Check sheet for the modelled part. Datum: model origin and axes. Units: mm. A direction names the side the tool comes from. Give positions to 0.01 mm unless a question says otherwise; leave off trailing zeros. Order: outer loops, then holes, each group sorted by start corner. A loop starts at its lowest first (then second) coordinate and runs counter-clockwise, first axis right, second up.
Item 1: Access from +Z, -Z, +X, -X, +Y, -Y to the whole of each face (thin tool, end or side, straight path). Record for faces 4 (the cylindrical face through (889.127, 47.139, -61.478)), 5 (the cylindrical face through (884.46, -24.22, 76.92)).
Item 2: Sectioned sample at A-A on x = 840. Record the boundary of the cut face in (y, z) (3 decimals).
Item 3: Release check for a two-part mould opening along Z. For faces 1 (the conical face through (109.73, 12.52, -2.78)), 2 (the flat face through (95.684, 9, 9)), 3 (the conical face through (1042.485, 75.822, -16.837)) record: released by +Z, released by -Z, zero draft, split by the parting line, or undercut.
Item 4: Gauge pin test, flat ends, axial feed: P1, Ø2, axis at x = 698.5, y = -44.5, coming from the -Z side; P2, Ø1.5, axis at x = 402, z = 34.5, coming from the +Y side; P3, Ø1.5, axis at x = 945.5, y = 62.5, coming from the -Z side. Record the tip position at first contact, or that the pin passes through.
Item 5: Material ranges on line 1 along Y through (x, z) = (861, 0) (3 decimals); line 2 along Z through (x, y) = (686, 61); line 3 along Y through (x, z) = (547.5, -42), recorded low to high.
from build123d import *

# Parameters (mm, degrees)
CHAMFER1_SIZE      = 16.51
SKETCH2_R          = 12.25
CUT_EXTRUDE1_DEPTH = 165


with BuildPart() as part:
    # Sketch1 → Revolve5 (revolve)
    with BuildSketch(Plane(origin=(0, 0, 0), x_dir=(1, 0, 0), z_dir=(0, 1, 0)), mode=Mode.PRIVATE) as revolve5_sk:
        with BuildLine():
            Line((98.225852671, 21.465396338), (95.684220755, 21.057997163))
            Line((95.684220755, 21.057997163), (95.684220755, 0))
            Line((95.684220755, 0), (98.726886962, 0))
            Line((98.726886962, 0), (98.726886962, 18.330178699))
            add(Edge.make_bspline(
                [(98.726886962, 18.330178699), (113.994878644, 20.770132881), (144.577764754, 25.330670583), (205.898051252, 33.589807316), (282.72017046, 42.680521232), (375.073984944, 52.176751592), (467.547747058, 60.469235877), (560.11629344, 67.637393605), (637.322841402, 72.653277734), (694.420933949, 75.753057643), (720.626011218, 76.995143626), (731.378470364, 77.47)],
                knots=[0.119456002, 0.119456002, 0.119456002, 0.119456002, 0.174490002, 0.229524002, 0.339592002, 0.449660001, 0.559728001, 0.669796001, 0.779864001, 0.834898, 0.873185267, 0.873185267, 0.873185267, 0.873185267], degree=3))
            Line((731.378470364, 77.47), (1042.519676327, 77.47))
            Line((1042.519676327, 77.47), (1041.959838164, 80.645))
            Line((1041.959838164, 80.645), (731.308396413, 80.645))
            add(Edge.make_bspline(
                [(98.225852671, 21.465396338), (124.397667511, 25.647873666), (176.884669485, 33.109736653), (282.119502984, 46.013248572), (413.979840243, 59.356838077), (572.506921448, 72.05625987), (678.351858694, 78.306302486), (731.308396413, 80.645)],
                knots=[0.119456002, 0.119456002, 0.119456002, 0.119456002, 0.213682547, 0.307909091, 0.496362181, 0.68481527, 0.873268359, 0.873268359, 0.873268359, 0.873268359], degree=3))
        make_face()
    revolve(revolve5_sk.sketch.rotate(Axis((0, 0, 0), (1, 0, 0)), 180), axis=Axis((0, 0, 0), (1, 0, 0)))

    # Chamfer1
    # the kernel refuses this chamfer: 19.899620903, 16.51 mm, written as the material it adds along each edge
    with BuildSketch(Plane(origin=(98.726886962, 0, 0), x_dir=(0, 0, 1), z_dir=(0, 1, 0))) as chamfer1_piece_1:
        with BuildLine():
            Line((18.330178699 - CHAMFER1_SIZE, 0), (21.36915573, 19.548977031))
            ThreePointArc((21.36915573, 19.548977031), (19.91924557, 10.088803652), (18.330178699, 0))
            Line((18.330178699, 0), (18.330178699 - CHAMFER1_SIZE, 0))
        make_face()
    revolve(axis=Axis((98.726886962, 0, 0), (1, 0, 0)))

    # Sketch2 → Cut-Extrude1 (cut)
    with BuildSketch(Plane.ZY.offset(-95.684220755)):
        Circle(SKETCH2_R)
    extrude(amount=-CUT_EXTRUDE1_DEPTH, mode=Mode.SUBTRACT)


solid = part.part
Report:
1. face 4: +X
1. face 5: +X, -X
2. outline: circle Ø161.29 at (0, 0); hole circle Ø154.94 at (0, 0)
3. face 1: undercut
3. face 2: zero draft
3. face 3: split by the parting line
4. P1: stops at z = -66.06
4. P2: stops at y = 46.81
4. P3: stops at z = -51.87
5. line 1: y = -80.645 to -77.47, 77.47 to 80.645
5. line 2: z = -49.34 to -44.1, 44.1 to 49.34
5. line 3: y = -55.65 to -51.6, 51.6 to 55.65
